from build123d import *

# Parameters (mm, degrees)
SKETCH1_W           = 1800
SKETCH1_H           = 850
BOSS_EXTRUDE1_DEPTH = 7.5
CUT_EXTRUDE1_DEPTH  = 480
FILLET1_R           = 20


with BuildPart() as part:
    # Sketch1 → Boss-Extrude1 (new, symmetric)
    with BuildSketch(Plane(origin=(0, 0, 0), x_dir=(1, 0, 0), z_dir=(0, 1, 0))):
        Rectangle(SKETCH1_W, SKETCH1_H)
    extrude(amount=BOSS_EXTRUDE1_DEPTH, both=True)

    # Sketch2 → Cut-Extrude1 (cut)
    with BuildSketch(Plane(origin=(0, 7.5, 0), x_dir=(1, 0, 0), z_dir=(0, 1, 0))):
        Polygon((-300, 390), (300, 390), (100, -390), (-108, -390), align=None)
    extrude(amount=-CUT_EXTRUDE1_DEPTH, mode=Mode.SUBTRACT)

    # Fillet1
    fillet1_edges = [part.edges().sort_by_distance(p)[0] for p in [
        (-108, 0, 390),
        (-300, 0, -390),
        (300, 0, -390),
        (100, 0, 390),
    ]]
    fillet(fillet1_edges, radius=FILLET1_R)


solid = part.part
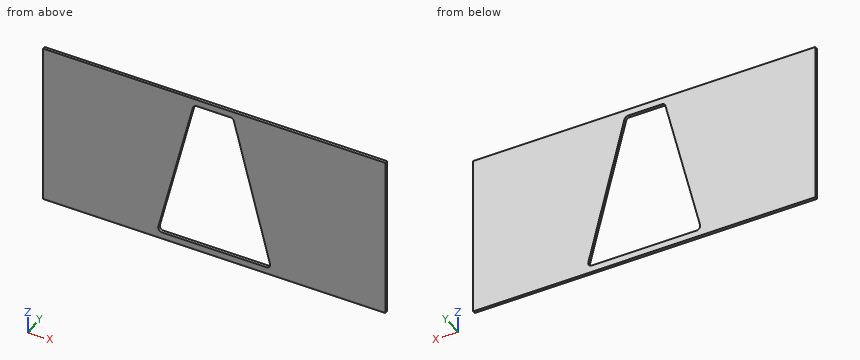
Verification items for the finished model (mm, model axes). Coordinates: 2 decimals unless noted, no trailing zeros. Write each loop counter-clockwise with the first axis right and the second up, starting at its lowest first coordinate (ties: lowest second). Pieces come first, ordered by that corner, then holes. Notation, with made-up numbers: (82, 26.5) -> (133, 26.5) arc R15 ccw to (133, 46.5) -> close; hole circle Ø1 at (78.25, -37). An arc over 180 degrees is marked (long way). One line per item, written item: value. Start each with the question number.
Q1. Thickness scan on L1, parallel to X at y = -0.5, z = -370; L2, parallel to X at y = -4.5, z = -192. Record the ranges inside material, lowest first. Write a range as from..to.
Q2. Cross-section at A-A on y = -4.5. Enter the section's corners in (x, z).
Q3. Cross-section at B-B on x = 17. Enter the section's corners in (y, z), and give its area (3 significant figures).
Q4. Cross-section at C-C on z = 275. Enter the section's corners in (x, y), and give its area (3 significant figures).
Checked values:
1. L1: x = -900..-294.48, 294.22..900
1. L2: x = -900..-251.26, 249.23..900
2. outline: (-900, -425) -> (900, -425) -> (900, 425) -> (-900, 425) -> close; hole (-293.9, -365.22) arc R20 ccw to (-274.48, -390) -> (274.22, -390) arc R20 ccw to (293.6, -365.03) -> (103.85, 374.97) arc R20 ccw to (84.48, 390) -> (-92.33, 390) arc R20 ccw to (-111.75, 374.78) -> close
3. outline: (-7.5, -425) -> (7.5, -425) -> (7.5, -390) -> (-7.5, -390) -> close; (-7.5, 390) -> (7.5, 390) -> (7.5, 425) -> (-7.5, 425) -> close
3. area: 1,050 mm²
4. outline: (-900, -7.5) -> (-136.31, -7.5) -> (-136.31, 7.5) -> (-900, 7.5) -> close; (129.49, -7.5) -> (900, -7.5) -> (900, 7.5) -> (129.49, 7.5) -> close
4. area: 23,000 mm²
